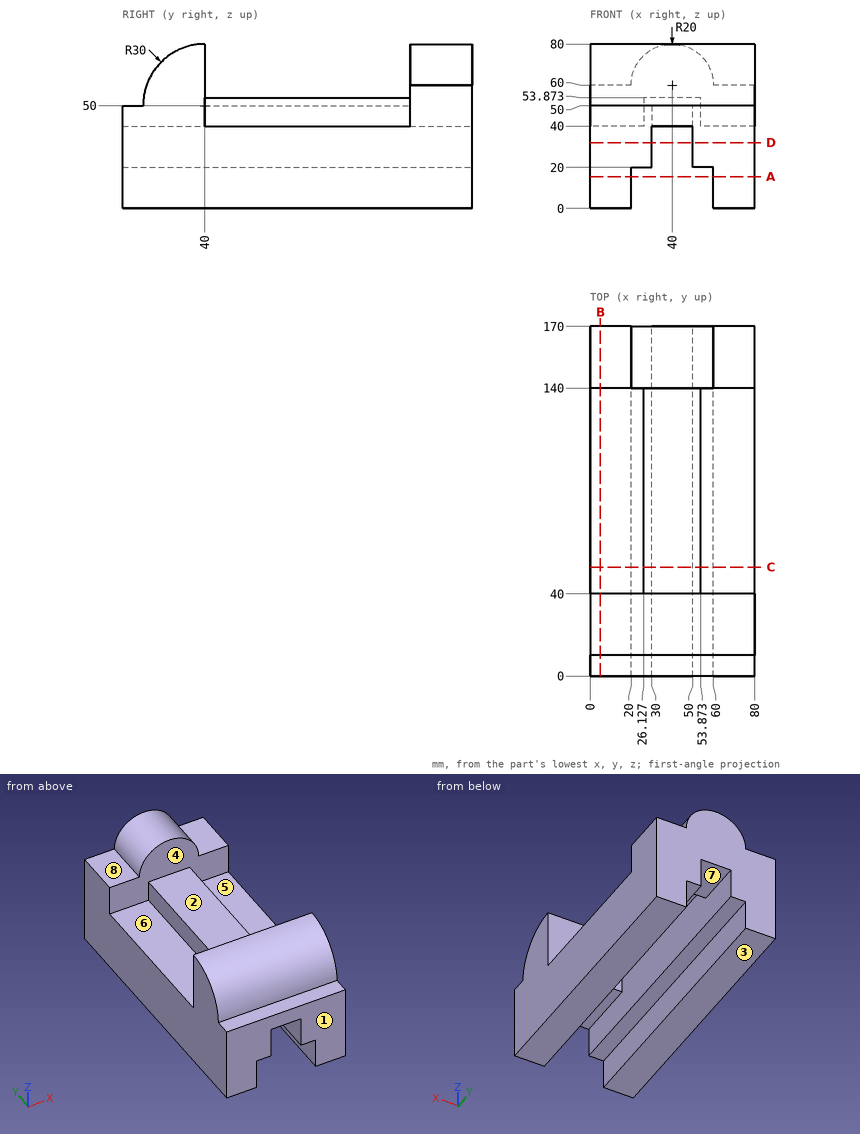
Here's the drawing with two shaded views (mm, measured from the low corner). I have some questions. A direction names the side the tool comes from. Round coordinates to 2 decimals unless told otherwise and drop trailing zeros. Loops run counter-clockwise (first coordinate to the right, second up) from the corner with the lowest first, then second, coordinate; pieces in that order, holes last.
Item 1: If we mould it in two halves opening along Y, with no side actions, what happens to the marked faces 1, 2 and 3? For each: +Y half, -Y half, draft (parallel to the pull), parting line (faces both ways), or undercut.
Item 2: Suppose I cut it at A-A, the plane z = 15.5. Write out the boundary of the cut face in (x, y).
Item 3: Which directions (+Z, -Z, +X, -X, +Y, -Y) give clear straight access to the entire face, cutting with the end or side of a thin tool? Please do the marked faces 4, 5, 6, 7 and 8.
Item 4: Suppose I cut it at C-C, the plane y = 53. Write out the boundary of the cut face in (x, z), then the cut area to 4 significant figures.
Item 5: Suppose I cut it at B-B, the plane x = 5. Write out the boundary of the cut face in (y, z).
Item 6: Please list where these lines run through material, in increasing order: L1, parallel to X at y = 57, z = 16.5; L2, parallel to Y at x = 34, z = 45; L3, parallel to X at y = 87, z = 27.5.
Item 7: Will these pins go through, and if not, where does the flat tip stop? pin 1 Ø1 at (y, z) = (81.5, 30) entering from -X; pin 2 Ø11 at (x, y) = (26, 52.5) entering from -Z; pin 3 Ø1.5 at (y, z) = (119.5, 50.5) entering from +X; pin 4 Ø3 at (y, z) = (152, 66.5) entering from +X (3 decimals).
Item 8: Suppose I cut it at D-D, the plane z = 32. Write out the boundary of the cut face in (x, y).
Reported:
1. face 1: -Y half
1. face 2: undercut
1. face 3: draft
2. outline: (0, 0) - (20, 0) - (20, 170) - (0, 170) - close; (60, 0) - (80, 0) - (80, 170) - (60, 170) - close
3. face 4: +Z
3. face 5: +Z, +X
3. face 6: +Z, -X
3. face 7: -Z, +Y, -Y
3. face 8: +Z, -X, +Y
4. outline: (0, 0) - (20, 0) - (20, 20) - (30, 20) - (30, 50) - (50, 50) - (50, 20) - (60, 20) - (60, 0) - (80, 0) - (80, 40) - (53.87, 40) - (53.87, 53.87) - (26.13, 53.87) - (26.13, 40) - (0, 40) - close
4. area: 2,185 mm2
5. outline: (0, 0) - (170, 0) - (170, 60) - (140, 60) - (140, 40) - (40, 40) - (40, 80) arc R30 ccw to (10, 50) - (0, 50) - close
6. L1: x = 0 to 20, 60 to 80
6. L2: y = 0 to 40, 140 to 170
6. L3: x = 0 to 30, 50 to 80
7. pin 1: stops at x = 0
7. pin 2: stops at z = 20
7. pin 3: stops at x = 53.87
7. pin 4: stops at x = 59.365
8. outline: (0, 0) - (30, 0) - (30, 170) - (0, 170) - close; (50, 0) - (80, 0) - (80, 170) - (50, 170) - close
